Design review of the part shown in the three views and the two pictorial views. Dimensions are in mm from the part's minimum x, y and z. A direction names the side the tool comes from. Round coordinates to 2 decimals unless told otherwise and drop trailing zeros. Loops run counter-clockwise (first coordinate to the right, second up) from the corner with the lowest first, then second, coordinate; pieces in that order, holes last. Notation, with made-up numbers: M 25,3.25 L 84,3.25 A25 cw 84,35.25 Z; hole C 42.25,8 d1. An arc over 180 degrees is marked long. Return JSON: item names as keys, results as strings. Group by question number.
Q1. Draft analysis for pull direction X (two halves, no side actions). For the marked faces 5, 6 and 7, state which applies: pulls with the +X half, pulls with the -X half, needs draft (parallel to the pull), parting line crosses it, or undercut.
Q2. To check wall thickness, follow line 1 along X through (y, z) = (5, 19.75); line 2 along X through (y, z) = (4.75, 2.25); line 3 along Y through (x, z) = (31.5, 12.5). State the ranges of each line that lie inside material, in increasing order.
Q3. For the marked faces 1, 2, 3 and 4, list the 3-axis set-ups (+Z, -Z, +X, -X, +Y, -Y) from which the entire face can be reached by the end or side of a thin tool; tool diameter is ignored.
Q4. Consider section B-B (x = 11.5). State the section outline as (y, z) points.
Q5. Consider section D-D (x = 17.5). State the section outline as (y, z) points, and give its area (3 significant figures).
Q6. Consider section A-A (z = 10.25). State the section outline as (x, y) points.
Q7. Clearance check with flat-ended pins moving along their axes: pin 1 Ø1.5 at (x, z) = (29.5, 11.5) entering from -Y; pin 2 Ø2.5 at (y, z) = (2.5, 13.5) entering from +X; pin 3 Ø1.5 at (x, y) = (1.5, 2.5) entering from +Z; pin 4 Ø0.9 at (x, y) = (11.5, 2.5) entering from +Z. State where each tip first meets the part, or that it passes through.
Q8. Consider section C-C (y = 3.45). Count the separate pieces of the cut face and the enclosed holes in it, and give its area (3 significant figures).
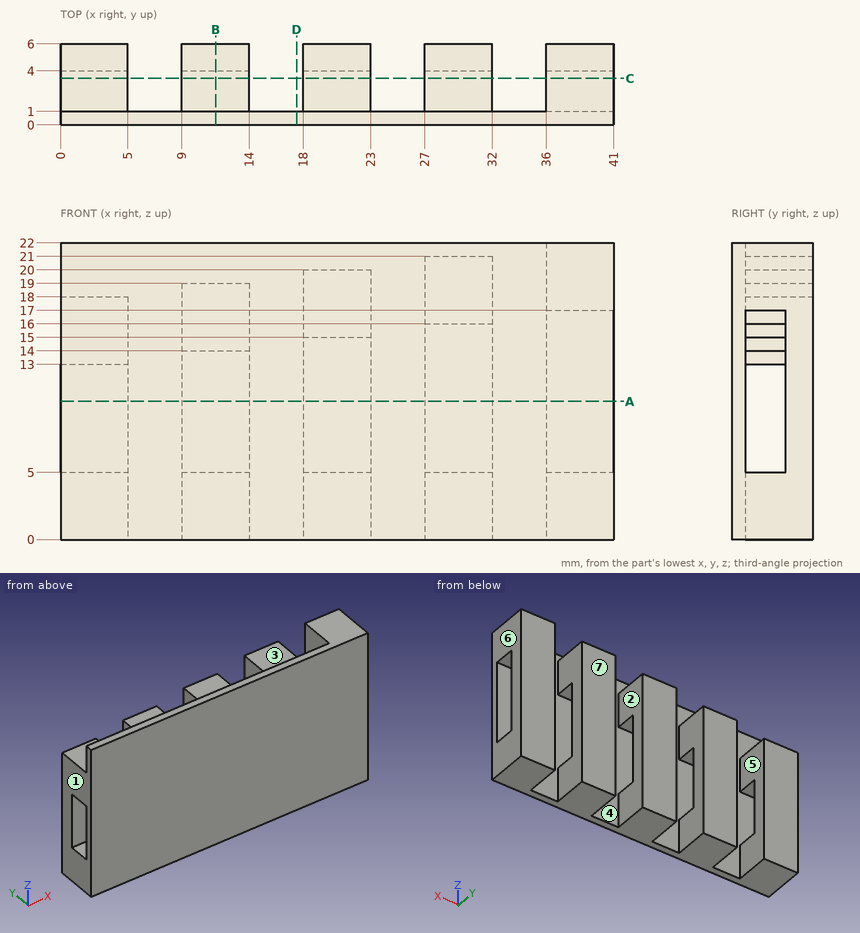
Values:
{
 "1": {"face 5": "undercut", "face 6": "pulls with the +X half", "face 7": "needs draft"},
 "2": {"line 1": "x = 18 to 23, 27 to 32, 36 to 41", "line 2": "x = 0 to 5, 9 to 14, 18 to 23, 27 to 32, 36 to 41", "line 3": "y = 0 to 1, 4 to 6"},
 "3": {"face 1": "+Z, -Z, -X, +Y, -Y", "face 2": "+Z, -Z, +Y", "face 3": "+Z, -X, +Y", "face 4": "none"},
 "4": {"outline": "M 0,0 L 6,0 L 6,19 L 1,19 L 1,22 L 0,22 Z; hole M 1,5 L 4,5 L 4,14 L 1,14 Z"},
 "5": {"outline": "M 0,0 L 1,0 L 1,22 L 0,22 Z", "area": "22.0 mm2"},
 "6": {"outline": "M 0,0 L 41,0 L 41,1 L 0,1 Z; M 0,4 L 5,4 L 5,6 L 0,6 Z; M 9,4 L 14,4 L 14,6 L 9,6 Z; M 18,4 L 23,4 L 23,6 L 18,6 Z; M 27,4 L 32,4 L 32,6 L 27,6 Z; M 36,4 L 41,4 L 41,6 L 36,6 Z"},
 "7": {"pin 1": "stops at y = 0", "pin 2": "stops at x = 14", "pin 3": "stops at z = 18", "pin 4": "stops at z = 19"},
 "8": {"separate pieces": "10", "enclosed holes": "0", "area": "250 mm2"}
}
